Input: part model. Units: mm. Frame: model coordinates. Coordinates: 2 decimals unless noted, no trailing zeros. Loops run counter-clockwise (first coordinate to the right, second up) from the corner with the lowest first, then second, coordinate; pieces in that order, holes last. Notation, with made-up numbers: (40, -33) - (89, -33) arc R23 cw to (89, -17) - close; hole circle Ø2 at (26.5, 4). An arc over 180 degrees is marked (long way). Use one line per item in the form item = value.
from build123d import *

# Parameters (mm, degrees)
SKETCH1_W           = 50.8
SKETCH1_H           = 76.2
BOSS_EXTRUDE1_DEPTH = 4.203048037
SKETCH3_R           = 11.1252
SKETCH3_R_2         = 12.7
CUT_EXTRUDE1_DEPTH  = 92.677399684
FILLET2_R           = 12.7


with BuildPart() as part:
    # Sketch1 → Boss-Extrude1 (new body)
    with BuildSketch(Plane.YZ):
        with Locations((25.4, 38.1)):
            Rectangle(SKETCH1_W, SKETCH1_H)
    extrude(amount=BOSS_EXTRUDE1_DEPTH)

    # Sketch3 → Cut-Extrude1 (cut, through all)
    with BuildSketch(Plane.YZ.offset(4.203048037)):
        with Locations(Location((25.4, 57.15, 0), (0, 0, 270))):
            Circle(SKETCH3_R)
        with Locations(Location((25.4, 19.05, 0), (0, 0, 270))):
            Circle(SKETCH3_R_2)
    extrude(amount=-CUT_EXTRUDE1_DEPTH, mode=Mode.SUBTRACT)

    # Fillet2
    fillet2_edges = [part.edges().sort_by_distance(p)[0] for p in [
        (2.101524019, 0, 0),
        (2.101524019, 0, 76.2),
        (2.101524019, 50.8, 76.2),
        (2.101524019, 50.8, 0),
    ]]
    fillet(fillet2_edges, radius=FILLET2_R)


solid = part.part
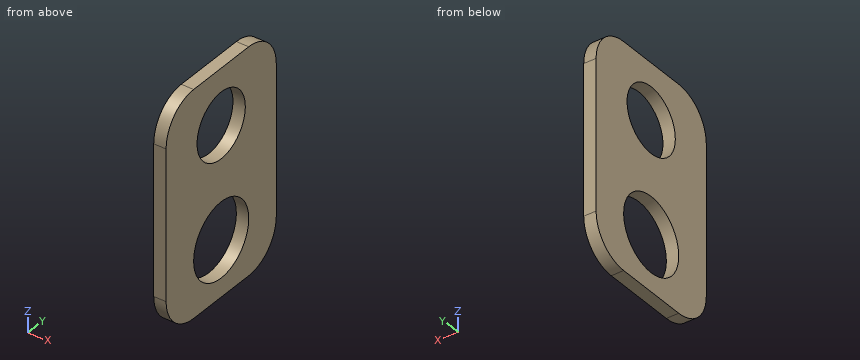
Q1. Cut plane D-D, the plane z = 19.05. Return loops of the section in (x, y).
Check values:
outline = (0, 0) - (4.2, 0) - (4.2, 12.7) - (0, 12.7) - close; (0, 38.1) - (4.2, 38.1) - (4.2, 50.8) - (0, 50.8) - close
Q2. Cut plane C-C, the plane x = 2.6. Return loops of the section in (y, z).
Check values:
outline = (0, 12.7) arc R12.7 ccw to (12.7, 0) - (38.1, 0) arc R12.7 ccw to (50.8, 12.7) - (50.8, 63.5) arc R12.7 ccw to (38.1, 76.2) - (12.7, 76.2) arc R12.7 ccw to (0, 63.5) - close; hole circle Ø25.4 at (25.4, 19.05); hole circle Ø22.25 at (25.4, 57.15)
Q3. Cut plane A-A, the plane z = 57.15. Return loops of the section in (x, y).
Check values:
outline = (0, 0) - (4.2, 0) - (4.2, 14.27) - (0, 14.27) - close; (0, 36.53) - (4.2, 36.53) - (4.2, 50.8) - (0, 50.8) - close
Q4. Ray query, line 1 along Y through (x, z) = (2.85, 57.15); line 2 along Z through (x, y) = (2.3, 17); line 3 along Z through (x, y) = (1.65, 19.5). Return the intervals inside material, ascending. Write a range as [from, to].
Check values:
line_1 = [0, 14.27], [36.53, 50.8]
line_2 = [0, 9.52], [28.58, 49.86], [64.44, 76.2]
line_3 = [0, 7.8], [30.3, 47.72], [66.58, 76.2]
Q5. First-contact query: P1, Ø1, axis at x = 3, y = 11, coming from the +Z side; P2, Ø1, axis at x = 2, y = 44, coming from the -Z side. Flat tips, straight axial feed; report the tip coordinate or a pass-through.
Check values:
P1 = 76.14
P2 = 1.21
Q6. Cut plane B-B, the plane y = 25.4. Return loops of the section in (x, z).
Check values:
outline = (0, 0) - (4.2, 0) - (4.2, 6.35) - (0, 6.35) - close; (0, 31.75) - (4.2, 31.75) - (4.2, 46.02) - (0, 46.02) - close; (0, 68.28) - (4.2, 68.28) - (4.2, 76.2) - (0, 76.2) - close
